from build123d import *

# Parameters (mm, degrees)
CROSSRECESS_DEPTH = 0.825
DRAFT9_ANGLE      = 30
FILLET5_R         = 0.3
LPATTERN10_COUNT  = 10
LPATTERN10_PITCH  = 0.3246


with BuildPart() as part:
    # Sketch1 → Base (revolve)
    with BuildSketch(Plane.XY, mode=Mode.PRIVATE) as base_sk:
        Polygon((5, 1.5), (2.65, 1.5), (1.65, 1.5), (0.55, 2.6), (0, 2.6), (0, 0), (5, 0), align=None)
    revolve(base_sk.sketch.rotate(Axis((4.515812911, 0, 0), (-1, 0, 0)), 90), axis=Axis((4.515812911, 0, 0), (-1, 0, 0)))

    # Sketch6 → CrossRecess (cut)
    with BuildSketch(Plane(origin=(0, 0, 0), x_dir=(0, 0, -1), z_dir=(1, 0, 0))):
        Polygon((0.32, 0.32), (0.32, 1.6), (-0.32, 1.6), (-0.32, 0.32), (-1.6, 0.32), (-1.6, -0.32), (-0.32, -0.32), (-0.32, -1.6), (0.32, -1.6), (0.32, -0.32), (1.6, -0.32), (1.6, 0.32), align=None)
    extrude(amount=CROSSRECESS_DEPTH, mode=Mode.SUBTRACT)

    # Draft9
    draft9_faces = [part.faces().sort_by_distance(p)[0] for p in [
        (0.4125, 1.6, 0),
        (0.4125, 0, 1.6),
        (0.4125, -1.6, 0),
        (0.4125, 0, -1.6),
    ]]
    draft(draft9_faces, Plane(origin=(0, 2.6, 0), x_dir=(0, 0, -1), z_dir=(-1, 0, 0)), DRAFT9_ANGLE)

    # Fillet5
    fillet5_edges = [part.edges().sort_by_distance(p)[0] for p in [
        (0.4125, 0.32, 0.32),
        (0.4125, -0.32, 0.32),
        (0.4125, -0.32, -0.32),
        (0.4125, 0.32, -0.32),
    ]]
    fillet(fillet5_edges, radius=FILLET5_R)

    # Sketch9 → Cut-Revolve10 (revolve, cut)
    with BuildSketch(Plane.XY, mode=Mode.PRIVATE) as cut_revolve10_sk:
        Polygon((5, 1.265740128), (5.13525, 1.5), (5.13525, 1.7705), (4.86475, 1.7705), (4.86475, 1.5), align=None)
    cut_revolve10 = revolve(cut_revolve10_sk.sketch.rotate(Axis((0, 0, 0), (1, 0, 0)), 270), axis=Axis((0, 0, 0), (1, 0, 0)), mode=Mode.SUBTRACT)

    # LPattern10: Cut-Revolve10 ×10
    with Locations(*[(-i * LPATTERN10_PITCH, 0, 0) for i in range(1, LPATTERN10_COUNT)]):
        add(cut_revolve10, mode=Mode.SUBTRACT)


solid = part.part
CAD build for the part. Positions are in the model's coordinates, mm. A direction names the side the tool comes from. Round coordinates to 2 decimals unless told otherwise and drop trailing zeros. Order: outer loops, then holes, each group sorted by start corner. A loop starts at its lowest first (then second) coordinate and runs counter-clockwise, first axis right, second up. Notation, with made-up numbers: (79, -37) -> (97, -37) arc R21 ccw to (97, -30) -> close; hole circle Ø8 at (-21.75, 22). An arc over 180 degrees is marked (long way). Write item = value, one per line. Start each with the question number.
(1) Pin check, flat tips, straight feed: P1, Ø0.9, axis at x = 0.5, z = 1, coming from the +Y side; P2, Ø2, axis at x = 3.5, z = 0.5, coming from the +Y side; P3, Ø0.9, axis at x = 0.5, z = 1, coming from the -Y side; P4, Ø2.5, axis at y = 0, z = 0, coming from the -X side. Stop position of each tip, or through.
(2) Probe line 1 (Y direction, x = 0.35, z = -0.1); line 2 (X direction, y = 0.8, z = 0.1) (3 decimals); line 3 (Z direction, x = 0.25, y = -1.1). List the from-to ranges inside material, lowest first. Write a range as [from, to].
(3) Which spindle directions (+Z, -Z, +X, -X, +Y, -Y) get a long thin tool onto all of the face, cutting with end or side? Do faces 1 (the flat face through (0.4, -1, -0.32)), 2 (the flat face through (5, 0, 0)). Say none if no direction does.
(4) Cut at A-A, the plane x = 1.35. List the corners of the cut face in (y, z), then the cut area to 3 significant figures.
Model answer:
q1.P1 = 2.54
q1.P2 = 1.5
q1.P3 = -2.54
q1.P4 = 0
q2.line_1 = [-2.6, -1.4], [1.4, 2.6]
q2.line_2 = [0.825, 5]
q2.line_3 = [-2.36, -0.32], [0.32, 2.36]
q3.face_1 = -X
q3.face_2 = +Z, -Z, +X, +Y, -Y
q4.outline = circle Ø3.6 at (0, 0)
q4.area = 10.2 mm2
